```python
from build123d import *

# Parameters (mm, degrees)
SKETCH_1_R          = 2
EXTRUDE_1_DEPTH     = 1.5
SKETCH_2_R          = 8
EXTRUDE_2_DEPTH     = 25
SKETCH_3_R          = 1.5
CUT_EXTRUDE_1_DEPTH = 2
SKETCH_4_R          = 6
CUT_EXTRUDE_2_DEPTH = 20
FILLET_5_R          = 0.5
FILLET_6_R          = 2


with BuildPart() as part:
    # 草图1 → 凸台-拉伸1 (new, symmetric)
    with BuildSketch(Plane.XY):
        with BuildLine():
            Line((0, 0), (6, 0))
            Line((6, 0), (6, 6))
            ThreePointArc((6, 6), (3, 9), (0, 6))
            Line((0, 6), (0, 0))
        make_face()
        with Locations((3, 6)):
            Circle(SKETCH_1_R, mode=Mode.SUBTRACT)
    extrude(amount=EXTRUDE_1_DEPTH, both=True)

    # 草图2 → 凸台-拉伸2 (add)
    with BuildSketch(Plane.XZ):
        with Locations(Location((3.022849102, 0, 0), (0, 0, 270))):
            Circle(SKETCH_2_R)
    extrude(amount=EXTRUDE_2_DEPTH)

    # 草图3 → 切除-拉伸1 (cut)
    with BuildSketch(Plane.XZ.offset(25)):
        with Locations(Location((2.994848376, 0, 0), (0, 0, 270))):
            Circle(SKETCH_3_R)
    extrude(amount=-CUT_EXTRUDE_1_DEPTH, mode=Mode.SUBTRACT)

    # 草图4 → 切除-拉伸2 (cut)
    with BuildSketch(Plane.XZ.offset(23)):
        with Locations(Location((2.994848376, 0, 0), (0, 0, 270))):
            Circle(SKETCH_4_R)
    extrude(amount=-CUT_EXTRUDE_2_DEPTH, mode=Mode.SUBTRACT)

    # 圆角5
    fillet_5_edges = [part.edges().sort_by_distance(p)[0] for p in [
        (6, 3, 1.5),
        (1, 6, -1.5),
        (1, 6, 1.5),
        (3, 9, 1.5),
        (0, 3, 1.5),
        (3, 9, -1.5),
        (6, 3, -1.5),
        (3, 0, -1.5),
        (0, 3, -1.5),
        (3, 0, 1.5),
        (6, 0, 0),
        (0, 0, 0),
    ]]
    fillet(fillet_5_edges, radius=FILLET_5_R - 0.0001)  # a hair under: the kernel refuses the full size

    # 圆角6
    fillet_6_edges = [part.edges().sort_by_distance(p)[0] for p in [
        (3.022849102, 0, 8),
    ]]
    fillet(fillet_6_edges, radius=FILLET_6_R)


solid = part.part
```
Can you work these out from the model? Positions are in its coordinate system, mm. A direction names the side the tool comes from. Give positions to 0.01 mm unless a question says otherwise; leave off trailing zeros. Loops run counter-clockwise (first coordinate to the right, second up) from the corner with the lowest first, then second, coordinate; pieces in that order, holes last. Notation, with made-up numbers: M 54,60.25 L 77,60.25 A13 ccw 77,84.25 Z; hole C 18,-36 d2. An arc over 180 degrees is marked long. Use one line per item in the form item = value. Start each with the question number.
(1) On a 3-axis mill with a long thin cutter (end or side, diameter ignored), from which of +Z, -Z, +X, -X, +Y, -Y can I reach the whole of each face in a straight line? I mean faces 1 (the cylindrical face through (4.26, -24.014, -0.806)), 2 (the flat face through (3, 3, -1.5)), 3 (the cylindrical face through (4.8, -13.14, -5.72)), 4 (the flat face through (3, 3, 1.5)), 5 (the flat face through (0, 3, 0)). Say none if no direction works.
(2) Please list where these lines run through material, in increasing order: line 1 (Y direction, x = 6.5, z = -1.5); line 2 (Y direction, x = 3, z = -0.35); line 3 (X direction, y = -23.95, z = 0).
(3) I want a section at B-B, the plane y = 2. Write out the boundary of the cut face in (x, z), and give its area (3 significant figures).
(4) I want a section at A-A, the plane z = 0. Write out the boundary of the cut face in (x, y).
(5) Thinking about a two-plate mould opening in X: for faces 6 (the flat face through (6, 3, 0)), 7 (the flat face through (1.7, -23, -1.2)), 8 (the cylindrical face through (-4.787, -13.339, 1.734)), which applies, released by +X, released by -X, zero draft, split by the parting line, or undercut?
(6) I'm going to push flat-ended pins straight in: P1, Ø2, axis at y = 4.5, z = 0.5, coming from the +X side; P2, Ø2.5, axis at x = 3, y = 4, coming from the +Z side; P3, Ø5.5, axis at x = 2.5, y = 5, coming from the -Z side. Where does each tip first touch, or does it pass through?
(7) I want a section at C-C, the plane y = -13. Write out the boundary of the cut face in (x, z), and give its area (3 significant figures).
Worked out:
q1.face_1 = -Y
q1.face_2 = -Z, +X, -X, +Y
q1.face_3 = none
q1.face_4 = +Z, +X, -X, +Y
q1.face_5 = +Z, -Z, -X, +Y
q2.line_1 = -25 to -23, -3 to 0
q2.line_2 = -3 to 4, 8 to 9
q2.line_3 = -4.98 to 1.49, 4.49 to 11.02
q3.outline = M 0,-1 A0.5 ccw 0.5,-1.5 L 5.5,-1.5 A0.5 ccw 6,-1 L 6,1 A0.5 ccw 5.5,1.5 L 0.5,1.5 A0.5 ccw 0,1 Z
q3.area = 17.8 mm²
q4.outline = M -4.98,-25 L 1.49,-25 L 1.49,-23 L -3.01,-23 L -3.01,-3 L 8.99,-3 L 8.99,-23 L 4.49,-23 L 4.49,-25 L 11.02,-25 L 11.02,-2 A2 ccw 9.02,0 L 6.5,0 A0.5 cw 6,0.5 L 6,6 A3 ccw 0,6 L 0,0.5 A0.5 cw -0.5,0 L -2.98,0 A2 ccw -4.98,-2 Z; hole C 3,6 d4
q5.face_6 = released by +X
q5.face_7 = undercut
q5.face_8 = split by the parting line
q6.P1 = 6
q6.P2 = 1.5
q6.P3 = -1.5
q7.outline = C 3.02,0 d16; hole C 2.99,0 d12
q7.area = 88.0 mm²
